Job drawing, mm, ordinate dimensions from the low corner. One solid piece. Round coordinates to 2 decimals unless told otherwise and drop trailing zeros. Write each loop counter-clockwise with the first axis right and the second up, starting at its lowest first coordinate (ties: lowest second). Pieces come first, ordered by that corner, then holes.
1) Flat gauge pin, fed straight in: pin 1 (3 mm diameter, centred on x = 11, y = 22, fed in from -Z). Where does the tip first touch, or does it go through?
2) Pull direction Y, two halves, no side cores. Call the marked faces 1, 2 and 3: +Y half, -Y half, draft (parallel to the pull), parting line (faces both ways), or undercut.
3) Saw through at A-A on x = 14. Write the cut outline in (y, z).
4) Saw through at B-B on z = 5.25. Write the cut outline in (x, y).
5) Saw through at C-C on y = 9. Write the cut outline in (x, z).
6) Saw through at D-D on x = 24.5. Write the cut outline in (y, z).
7) Drill centre lines: L1, parallel to Y at x = 14, z = 3.75; L2, parallel to X at y = 10.5, z = 3.75 (1 decimal); L3, parallel to Y at x = 15.25, z = 1.5. Where is each one in solid material? Low to high.
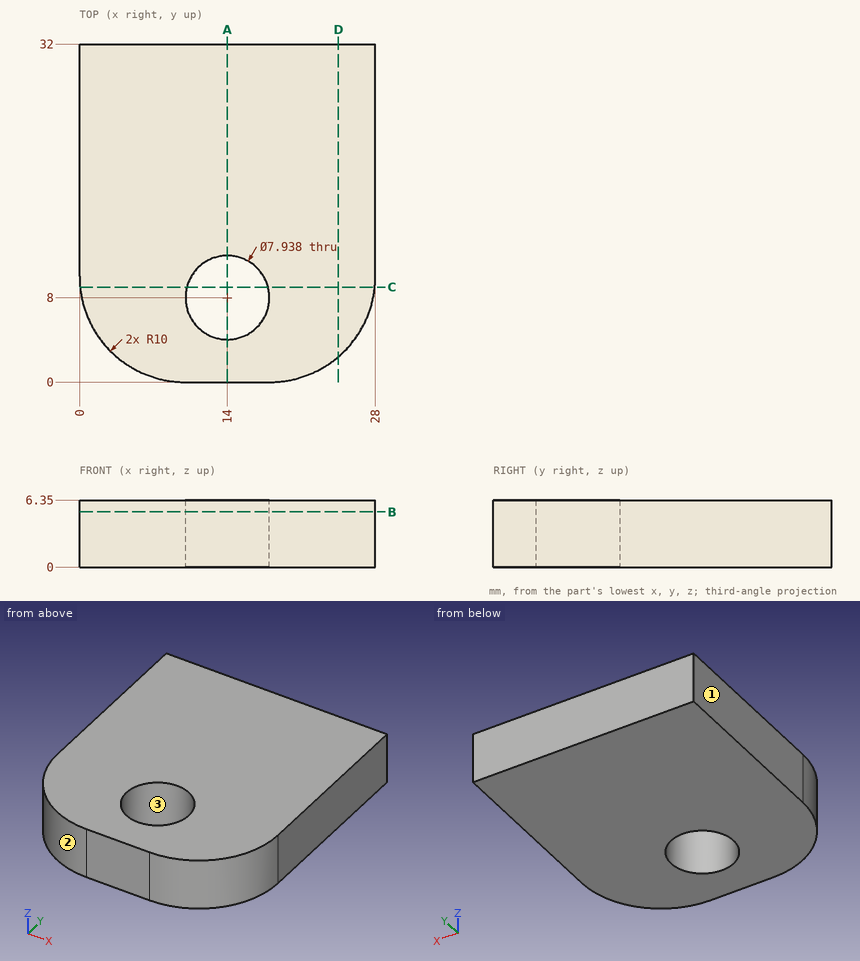
Completed:
1. pin 1: stops at z = 0
2. face 1: draft
2. face 2: -Y half
2. face 3: undercut
3. outline: (0, 0) - (4.03, 0) - (4.03, 6.35) - (0, 6.35) - close; (11.97, 0) - (32, 0) - (32, 6.35) - (11.97, 6.35) - close
4. outline: (0, 10) arc R10 ccw to (10, 0) - (18, 0) arc R10 ccw to (28, 10) - (28, 32) - (0, 32) - close; hole circle Ø7.94 at (14, 8)
5. outline: (0.05, 0) - (10.16, 0) - (10.16, 6.35) - (0.05, 6.35) - close; (17.84, 0) - (27.95, 0) - (27.95, 6.35) - (17.84, 6.35) - close
6. outline: (2.4, 0) - (32, 0) - (32, 6.35) - (2.4, 6.35) - close
7. L1: y = 0 to 4.03, 11.97 to 32
7. L2: x = 0 to 10.9, 17.1 to 28
7. L3: y = 0 to 4.23, 11.77 to 32
